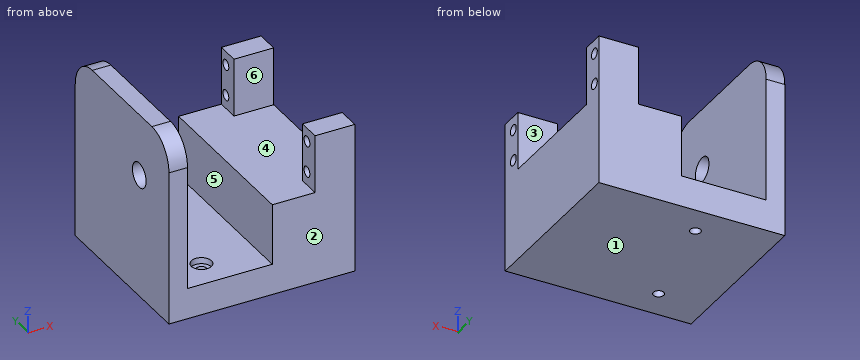
from build123d import *

# Parameters (mm, degrees)
ESQUISSE1_W                                          = 60
ESQUISSE1_H                                          = 55
BOSS_EXTRU_1_DEPTH                                   = 10
ESQUISSE2_W                                          = 6
ESQUISSE2_H                                          = 55
BOSS_EXTRU_2_DEPTH                                   = 50
ESQUISSE3_W                                          = 26.62
ESQUISSE3_H                                          = 55
BOSS_EXTRU_3_DEPTH                                   = 19.7
CHAMBRAGE_POUR_T_TE_CYLINDRIQUE_FENDUE_M_D           = 3.4
CHAMBRAGE_POUR_T_TE_CYLINDRIQUE_FENDUE_M_DEPTH       = 10
CHAMBRAGE_POUR_T_TE_CYLINDRIQUE_FENDUE_M_CBORE_D     = 6.5
CHAMBRAGE_POUR_T_TE_CYLINDRIQUE_FENDUE_M_CBORE_DEPTH = 2
CHAMBRAGE_POUR_T_TE_CYLINDRIQUE_FENDUE_M_TIP         = 1.021463052
CONG_1_R                                             = 10
ESQUISSE8_R                                          = 4
ENL_V_MAT_EXTRU_2_DEPTH                              = 6
ESQUISSE12_W                                         = 12.82
ESQUISSE12_H                                         = 7.4
BOSS_EXTRU_4_DEPTH                                   = 18.8
D_GAGEMENT_M32_D                                     = 3.4
D_GAGEMENT_M32_DEPTH                                 = 12.82
D_GAGEMENT_M32_TIP                                   = 1.021463052


with BuildPart() as part:
    # Esquisse1 → Boss.-Extru.1 (new body)
    with BuildSketch(Plane.XY):
        with Locations((30, 27.5)):
            Rectangle(ESQUISSE1_W, ESQUISSE1_H)
    extrude(amount=BOSS_EXTRU_1_DEPTH)

    # Esquisse2 → Boss.-Extru.2 (add)
    with BuildSketch(Plane.XY.offset(10)):
        with Locations((3, 27.5)):
            Rectangle(ESQUISSE2_W, ESQUISSE2_H)
    extrude(amount=BOSS_EXTRU_2_DEPTH)

    # Esquisse3 → Boss.-Extru.3 (add)
    with BuildSketch(Plane.XY.offset(10)):
        with Locations((46.69, 27.5)):
            Rectangle(ESQUISSE3_W, ESQUISSE3_H)
    extrude(amount=BOSS_EXTRU_3_DEPTH)

    # Chambrage pour tête cylindrique fendue M31
    with Locations(Plane.XY.offset(10)):
        with Locations((23.38, 45), (16, 10)):
            CounterBoreHole(CHAMBRAGE_POUR_T_TE_CYLINDRIQUE_FENDUE_M_D / 2, CHAMBRAGE_POUR_T_TE_CYLINDRIQUE_FENDUE_M_CBORE_D / 2, CHAMBRAGE_POUR_T_TE_CYLINDRIQUE_FENDUE_M_CBORE_DEPTH, depth=CHAMBRAGE_POUR_T_TE_CYLINDRIQUE_FENDUE_M_DEPTH)
            with Locations((0, 0, -(CHAMBRAGE_POUR_T_TE_CYLINDRIQUE_FENDUE_M_DEPTH + CHAMBRAGE_POUR_T_TE_CYLINDRIQUE_FENDUE_M_TIP / 2))):  # 118° drill point
                Cone(0, CHAMBRAGE_POUR_T_TE_CYLINDRIQUE_FENDUE_M_D / 2, CHAMBRAGE_POUR_T_TE_CYLINDRIQUE_FENDUE_M_TIP, mode=Mode.SUBTRACT)

    # Congé1
    cong_1_edges = [part.edges().sort_by_distance(p)[0] for p in [
        (3, 0, 60),
        (3, 55, 60),
    ]]
    fillet(cong_1_edges, radius=CONG_1_R)

    # Esquisse8 → Enlèv. mat.-Extru.2 (cut)
    with BuildSketch(Plane.ZY):
        with Locations((40, 17.4)):
            Circle(ESQUISSE8_R)
    extrude(amount=-ENL_V_MAT_EXTRU_2_DEPTH, mode=Mode.SUBTRACT)

    # Esquisse12 → Boss.-Extru.4 (add)
    with BuildSketch(Plane.XY.offset(29.7)):
        with Locations((53.59, 3.7)):
            Rectangle(ESQUISSE12_W, ESQUISSE12_H)
        with Locations((53.59, 51.3)):
            Rectangle(ESQUISSE12_W, ESQUISSE12_H)
    extrude(amount=BOSS_EXTRU_4_DEPTH)

    # Dégagement M32
    with Locations(Plane.ZY.offset(-47.18)):
        with Locations((44.1, 52.35), (34.1, 52.35), (44.1, 4.75), (34.1, 4.75)):
            Hole(D_GAGEMENT_M32_D / 2, depth=D_GAGEMENT_M32_DEPTH)
            with Locations((0, 0, -(D_GAGEMENT_M32_DEPTH + D_GAGEMENT_M32_TIP / 2))):  # 118° drill point
                Cone(0, D_GAGEMENT_M32_D / 2, D_GAGEMENT_M32_TIP, mode=Mode.SUBTRACT)


solid = part.part
Input: part model. Units: mm. Frame: model coordinates. Face numbers are marked on the shaded views. A direction names the side the tool comes from. Coordinates: 2 decimals unless noted, no trailing zeros. Loops run counter-clockwise (first coordinate to the right, second up) from the corner with the lowest first, then second, coordinate; pieces in that order, holes last.
Q1. Draft query along Y for the marked faces 1, 2 and 3. Return one class per face: +Y half, -Y half, draft (parallel to the pull), parting line (faces both ways), or undercut.
Q2. Cut plane C-C (x = 16). Output: boundary loops of the cut face in (y, z).
Q3. Set-up query: the marked faces 4, 5 and 6. Return all of +Z, -Z, +X, -X, +Y, -Y with unobstructed straight access to the full face (end or side cutting, diameter ignored); none if empty.
Q4. Cut plane D-D (z = 26.5). Output: boundary loops of the cut face in (x, y).
Q5. Contact query for flat-ended pins moving along their axis: pin 1 (3 mm diameter, centred on y = 28, z = 53, fed in from +X); pin 2 (13.5 mm diameter, centred on x = 25.5, y = 18, fed in from +Z); pin 3 (2 mm diameter, centred on x = 23.38, y = 45, fed in from -Z); pin 4 (5 mm diameter, centred on x = 16, y = 10, fed in from +Z). Output: stop coordinate, or through.
Q6. Material intervals for line 1 (Y direction, x = 53.75, z = 44.1); line 2 (X direction, y = 32, z = 28.5); line 3 (Y direction, x = 23.38, z = 8.85), sorted ascending.
Q7. Cut plane A-A (z = 34.1). Output: boundary loops of the cut face in (x, y), then the cut area to 3 significant figures.
Q8. Cut plane B-B (y = 17.4). Output: boundary loops of the cut face in (x, z).
Working result:
1. face 1: draft
1. face 2: -Y half
1. face 3: undercut
2. outline: (0, 0) - (8.3, 0) - (8.3, 8) - (6.75, 8) - (6.75, 10) - (0, 10) - close; (11.7, 0) - (55, 0) - (55, 10) - (13.25, 10) - (13.25, 8) - (11.7, 8) - close
3. face 4: +Z
3. face 5: +Z, +Y, -Y
3. face 6: +Z, +X
4. outline: (0, 0) - (6, 0) - (6, 55) - (0, 55) - close; (33.38, 0) - (60, 0) - (60, 55) - (33.38, 55) - close
5. pin 1: stops at x = 6
5. pin 2: stops at z = 10
5. pin 3: passes through
5. pin 4: stops at z = 8
6. line 1: y = 0 to 3.05, 6.45 to 7.4, 47.6 to 50.65, 54.05 to 55
6. line 2: x = 0 to 6, 33.38 to 60
6. line 3: y = 0 to 41.75, 48.25 to 55
7. outline: (0, 0) - (6, 0) - (6, 55) - (0, 55) - close; (47.18, 0) - (60, 0) - (60, 3.05) - (47.18, 3.05) - close; (47.18, 6.45) - (60, 6.45) - (60, 7.4) - (47.18, 7.4) - close; (47.18, 47.6) - (60, 47.6) - (60, 50.65) - (47.18, 50.65) - close; (47.18, 54.05) - (60, 54.05) - (60, 55) - (47.18, 55) - close
7. area: 433 mm2
8. outline: (0, 0) - (60, 0) - (60, 29.7) - (33.38, 29.7) - (33.38, 10) - (6, 10) - (6, 36) - (0, 36) - close; (0, 44) - (6, 44) - (6, 60) - (0, 60) - close
